Could you check a few things on this drawing? It's one solid part, dimensions in mm from its lowest x, y, z. Give positions to 0.01 mm unless a question says otherwise; leave off trailing zeros. Loops run counter-clockwise (first coordinate to the right, second up) from the corner with the lowest first, then second, coordinate; pieces in that order, holes last. Notation, with made-up numbers: M 74,50.25 L 117,50.25 A20 cw 117,83.25 Z; hole C 34.5,27 d1. An arc over 180 degrees is marked long. Answer as a JSON object with one key per item and string values.
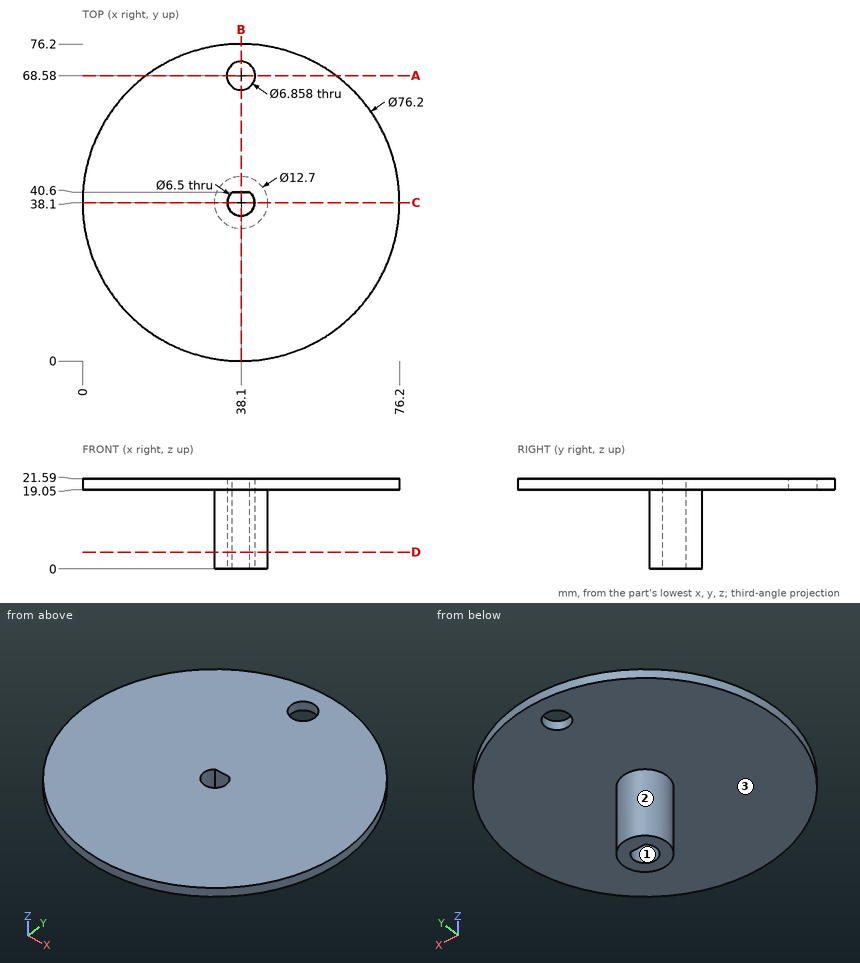
1) Suppose I cut it at B-B, the plane x = 38.1. Write out the boundary of the cut face in (y, z).
Answer list:
{"outline": "M 0,19.05 L 31.75,19.05 L 31.75,0 L 34.85,0 L 34.85,21.59 L 0,21.59 Z; M 40.6,0 L 44.45,0 L 44.45,19.05 L 65.15,19.05 L 65.15,21.59 L 40.6,21.59 Z; M 72.01,19.05 L 76.2,19.05 L 76.2,21.59 L 72.01,21.59 Z"}
2) Suppose I cut it at A-A, the plane y = 68.58. Write out the boundary of the cut face in (x, z).
Answer list:
{"outline": "M 15.24,19.05 L 34.67,19.05 L 34.67,21.59 L 15.24,21.59 Z; M 41.53,19.05 L 60.96,19.05 L 60.96,21.59 L 41.53,21.59 Z"}
3) Please list where these lines run through material, in increasing order: line 1 along Y through (x, z) = (38.1, 20.9); line 2 along Y through (x, z) = (38.1, 11.5); line 3 along Z through (x, y) = (30.5, 8). Write a range as from..to.
Answer list:
{"line 1": "0..34.85, 40.6..65.15, 72.01..76.2", "line 2": "31.75..34.85, 40.6..44.45", "line 3": "19.05..21.59"}
4) Will these pins go through, and if not, where does the flat tip stop? pin 1 Ø8 at (x, z) = (38, 14.5) entering from +Y; pin 2 Ø2 at (x, z) = (38, 6.5) entering from -Y; pin 3 Ø8 at (x, y) = (38.1, 68.58) entering from -Z.
Answer list:
{"pin 1": "y = 44.45", "pin 2": "y = 31.75", "pin 3": "z = 19.05"}
5) Suppose I cut it at C-C, the plane y = 38.1. Write out the boundary of the cut face in (x, z).
Answer list:
{"outline": "M 0,19.05 L 31.75,19.05 L 31.75,0 L 34.85,0 L 34.85,21.59 L 0,21.59 Z; M 41.35,0 L 44.45,0 L 44.45,19.05 L 76.2,19.05 L 76.2,21.59 L 41.35,21.59 Z"}
6) If we mould it in two halves opening along X, with no side actions, what happens to the marked faces 1, 2 and 3? For each: +X half, -X half, draft (parallel to the pull), parting line (faces both ways), or undercut.
Answer list:
{"face 1": "undercut", "face 2": "parting line", "face 3": "draft"}
7) Suppose I cut it at D-D, the plane z = 4. Write out the boundary of the cut face in (x, y).
Answer list:
{"outline": "C 38.1,38.1 d12.7; hole M 36.02,40.6 A3.25 ccw long 40.18,40.6 Z"}
